Verification items for the finished model (mm, model axes). Face numbers are marked on the shaded views. Give positions to 0.01 mm unless a question says otherwise; leave off trailing zeros. Put each result on its own line as item: value.
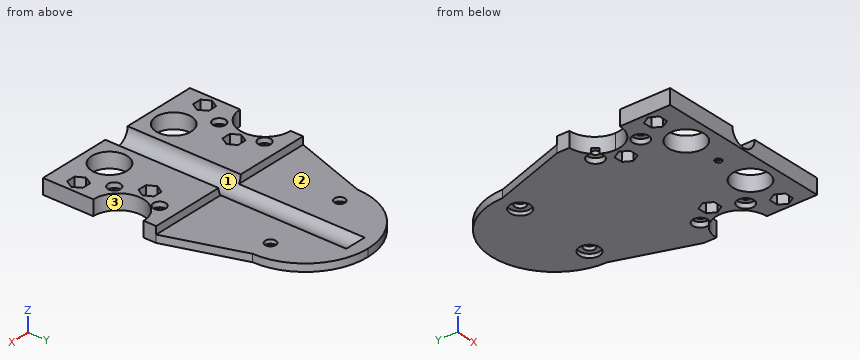
from build123d import *

# Parameters (mm, degrees)
SKETCH_1_R           = 1.3
EXTRUDE_1_DEPTH      = 6
SKETCH_1_3_R         = 2.1
EXTRUDE_2_DEPTH      = 3
SKETCH_3_R           = 5.3
CUT_EXTRUDE_1_DEPTH  = 95
SKETCH_6_R           = 3.2
SKETCH_6_R_2         = 3
CUT_EXTRUDE_3_DEPTH  = 2
SKETCH_9_R           = 4
CUT_EXTRUDE_6_DEPTH  = 1.5
CUT_EXTRUDE_7_DEPTH  = 4.0000001
CUT_EXTRUDE_8_DEPTH  = 7.0000001
SKETCH_12_R          = 7
CUT_EXTRUDE_9_DEPTH  = 7.0000001
SKETCH_13_R          = 2.5
CUT_EXTRUDE_11_DEPTH = 2


with BuildPart() as part:
    # Sketch 1 → Extrude 1 (new body)
    with BuildSketch(Plane.XY):
        Polygon((-35, 0), (0, 0), (35, 0), (35, 45), (0, 45), (-35, 45), align=None)
        Polygon((-26.420428959, 10.002120735), (-28.208377869, 6.901060912), (-31.78794891, 6.898940176), (-33.579571041, 9.997879265), (-31.791622131, 13.098939088), (-28.21205109, 13.101059824), align=None, mode=Mode.SUBTRACT)
        with Locations((-25, 20)):
            Circle(SKETCH_1_R, mode=Mode.SUBTRACT)
        Polygon((-16.420523373, 30.026084728), (-18.187671649, 26.913124673), (-21.767148276, 26.887039945), (-23.579476627, 29.973915272), (-21.812328351, 33.086875327), (-18.232851724, 33.112960055), align=None, mode=Mode.SUBTRACT)
        with Locations((-25, 38)):
            Circle(SKETCH_1_R, mode=Mode.SUBTRACT)
        with Locations((0, 10)):
            Circle(SKETCH_1_R, mode=Mode.SUBTRACT)
        Polygon((33.579530154, 10.017239862), (31.804695235, 6.908655884), (28.225165081, 6.891416023), (26.420469846, 9.982760138), (28.195304765, 13.091344116), (31.774834919, 13.108583977), align=None, mode=Mode.SUBTRACT)
        with Locations((25, 20)):
            Circle(SKETCH_1_R, mode=Mode.SUBTRACT)
        Polygon((23.579135684, 29.944133288), (21.74118585, 26.872444218), (18.162050166, 26.92831093), (16.420864316, 30.055866712), (18.25881415, 33.127555782), (21.837949834, 33.07168907), align=None, mode=Mode.SUBTRACT)
        with Locations((25, 38)):
            Circle(SKETCH_1_R, mode=Mode.SUBTRACT)
    extrude(amount=EXTRUDE_1_DEPTH)

    # Sketch 1_3 → Extrude 2 (add)
    with BuildSketch(Plane.XY):
        Polygon((0, 45), (35, 45), (35, 100), (-35, 100), (-35, 45), align=None)
        with Locations((-16.5, 75)):
            Circle(SKETCH_1_3_R, mode=Mode.SUBTRACT)
        with Locations((16.5, 75)):
            Circle(SKETCH_1_3_R, mode=Mode.SUBTRACT)
    extrude(amount=EXTRUDE_2_DEPTH)

    # Sketch 3 → Cut-Extrude 1 (cut)
    with BuildSketch(Plane(origin=(0, 0, 0), x_dir=(-1, 0, 0), z_dir=(0, -1, 0))):
        with Locations((0, -6)):
            Circle(SKETCH_3_R)
    extrude(amount=-CUT_EXTRUDE_1_DEPTH, mode=Mode.SUBTRACT)

    # Sketch 6 → Cut-Extrude 3 (cut)
    with BuildSketch(Plane(origin=(0, 0, 0), x_dir=(-1, 0, 0), z_dir=(0, 0, -1))):
        with Locations((25, 38)):
            Circle(SKETCH_6_R)
        with Locations((25, 20)):
            Circle(SKETCH_6_R)
        with Locations((-25, 20)):
            Circle(SKETCH_6_R)
        with Locations((-25, 38)):
            Circle(SKETCH_6_R_2)
    extrude(amount=-CUT_EXTRUDE_3_DEPTH, mode=Mode.SUBTRACT)

    # Sketch 9 → Cut-Extrude 6 (cut)
    with BuildSketch(Plane(origin=(0, 0, 0), x_dir=(-1, 0, 0), z_dir=(0, 0, -1))):
        with Locations((-16.5, 75)):
            Circle(SKETCH_9_R)
        with Locations((16.5, 75)):
            Circle(SKETCH_9_R)
    extrude(amount=-CUT_EXTRUDE_6_DEPTH, mode=Mode.SUBTRACT)

    # Sketch 10 → Cut-Extrude 7 (cut, through all)
    with BuildSketch(Plane.XY.offset(3)):
        with BuildLine():
            Line((-35, 45), (-25, 75))
            ThreePointArc((-25, 75), (-17.67766953, 92.67766953), (0, 100))
            Line((0, 100), (-35, 100))
            Line((-35, 100), (-35, 45))
        make_face()
        with BuildLine():
            Line((35, 100), (0, 100))
            ThreePointArc((0, 100), (17.67766953, 92.67766953), (25, 75))
            Line((25, 75), (35, 45))
            Line((35, 45), (35, 100))
        make_face()
    extrude(amount=-CUT_EXTRUDE_7_DEPTH, mode=Mode.SUBTRACT)

    # Sketch 11 → Cut-Extrude 8 (cut, through all)
    with BuildSketch(Plane.XY.offset(6)):
        with BuildLine():
            ThreePointArc((45, 30), (42.071067812, 37.071067812), (35, 40))
            Line((35, 40), (35, 30))
            Line((35, 30), (35, 20))
            ThreePointArc((35, 20), (42.071067812, 22.928932188), (45, 30))
        make_face()
        with BuildLine():
            Line((35, 30), (35, 40))
            ThreePointArc((35, 40), (25, 30), (35, 20))
            Line((35, 20), (35, 30))
        make_face()
        with BuildLine():
            ThreePointArc((-25, 30), (-27.928932188, 37.071067812), (-35, 40))
            Line((-35, 40), (-35, 30))
            Line((-35, 30), (-35, 20))
            ThreePointArc((-35, 20), (-27.928932188, 22.928932188), (-25, 30))
        make_face()
        with BuildLine():
            Line((-35, 30), (-35, 40))
            ThreePointArc((-35, 40), (-45, 30), (-35, 20))
            Line((-35, 20), (-35, 30))
        make_face()
    extrude(amount=-CUT_EXTRUDE_8_DEPTH, mode=Mode.SUBTRACT)

    # Sketch 12 → Cut-Extrude 9 (cut, through all)
    with BuildSketch(Plane.XY.offset(6)):
        with Locations((15.3, 10)):
            Circle(SKETCH_12_R)
        with Locations((-15.3, 10)):
            Circle(SKETCH_12_R)
    extrude(amount=-CUT_EXTRUDE_9_DEPTH, mode=Mode.SUBTRACT)

    # Sketch 13 → Cut-Extrude 11 (cut)
    with BuildSketch(Plane.XY.offset(6)):
        with Locations((-25, 20)):
            Circle(SKETCH_13_R)
        with Locations((25, 20)):
            Circle(SKETCH_13_R)
        with Locations((25, 38)):
            Circle(SKETCH_13_R)
        with Locations((-25, 38)):
            Circle(SKETCH_13_R)
    extrude(amount=-CUT_EXTRUDE_11_DEPTH, mode=Mode.SUBTRACT)


solid = part.part
Q1. Scan lines: line 1 along Y through (x, z) = (16.5, 2.2); line 2 along X through (y, z) = (5, 4.75); line 3 along Y through (x, z) = (18, 4.5). Record each from-to range of solid material in increasing order.
Answers follow:
line 1: y = 0 to 3.1, 16.9 to 29.91, 30.19 to 72.9, 77.1 to 93.78
line 2: x = -35 to -20.2, -10.4 to -5.15, 5.15 to 10.4, 20.2 to 35
line 3: y = 0 to 3.54, 16.46 to 27.22, 32.7 to 45
Q2. Go/stop test with flat-tipped pins: pin 1 Ø1.5 at (x, y) = (24, 39) entering from +Z; pin 2 Ø1.5 at (x, z) = (15.5, 2) entering from +Y; pin 3 Ø1.9 at (x, y) = (-25, 21) entering from -Z; pin 4 Ø1.5 at (x, z) = (-4, 4.5) entering from +Y. Record where each tip stops, or that it passes through.
Answers follow:
pin 1: stops at z = 4
pin 2: stops at y = 95.19
pin 3: stops at z = 2
pin 4: passes through
Q3. Release check for a two-part mould opening along X. For the marked faces 1, 2 and 3 record: released by +X, released by -X, zero draft, split by the parting line, or undercut.
Answers follow:
face 1: undercut
face 2: zero draft
face 3: released by +X
